Input: part model. Units: mm. Frame: model coordinates. A direction names the side the tool comes from. Give positions to 0.01 mm unless a question says otherwise; leave off trailing zeros. Write each loop counter-clockwise with the first axis right and the second up, starting at its lowest first coordinate (ties: lowest second). Pieces come first, ordered by that corner, then holes. Notation, with made-up numbers: (69, 2.5) - (82, 2.5) arc R18 cw to (82, 20.5) - close; hole circle Ø2 at (43, 1). An arc over 180 degrees is marked (long way). Answer as a JSON object with one key per item and string values. Group by question number.
Autodesk Inventor part; units mm, degrees
ref_plane "YZ Plane" through (0, 0, 0) normal (1, 0, 0) x (0, 1, 0)
ref_plane "XZ Plane" through (0, 0, 0) normal (0, 1, 0) x (-1, 0, 0)
ref_plane "XY Plane" through (0, 0, 0) normal (0, 0, 1) x (1, 0, 0)
sketch "Szkic1" plane through (0, 0, 0) normal (1, 0, 0) x (0, 1, 0)
  line L0 (3.5782, 14) -> (0.5782, 14)
  line L1 (0.5782, 14) -> (0.5782, 23)
  line L2 (0.5782, 23) -> (26.5782, 23)
  arc A0 (49.5782, 0) -> (26.5782, 23) centre (26.5782, 0) ccw
  line L3 (3.5782, 14) -> (3.5782, 18)
  line L4 (3.5782, 18) -> (26.5782, 18)
  arc A1 (44.5782, 0) -> (26.5782, 18) centre (26.5782, 0) ccw
  line L5 (3.5782, -14) -> (0.5782, -14)
  line L6 (0.5782, -14) -> (0.5782, -23)
  line L7 (0.5782, -23) -> (26.5782, -23)
  arc A2 (26.5782, -23) -> (49.5782, 0) centre (26.5782, 0) ccw
  line L8 (3.5782, -14) -> (3.5782, -18)
  line L9 (3.5782, -18) -> (26.5782, -18)
  arc A3 (26.5782, -18) -> (44.5782, 0) centre (26.5782, 0) ccw
  line L10 (51.5782, 6.5) -> (44.5782, 6.5)
  line L11 (44.5782, 6.5) -> (44.5782, -6.5)
  line L12 (44.5782, -6.5) -> (51.5782, -6.5)
  line L13 (54.5782, -3.5) -> (54.5782, 3.5)
  arc A4 (54.5782, 3.5) -> (51.5782, 6.5) centre (51.5782, 3.5) ccw
  arc A5 (51.5782, -6.5) -> (54.5782, -3.5) centre (51.5782, -3.5) ccw
  point P0 (0, 0)
  point P1 (2.0782, 14)
  point P2 (3.5782, 16)
  point P3 (2.0782, -14)
  point P4 (0.5782, 18.5)
  point P5 (48.6406, -6.5)
  point P6 (48.6406, 6.5)
  dimension "d0" = 9
  dimension "d2" = 5
  dimension "d3" = 3
  dimension "d4" = 23
  dimension "d5" = 14
  dimension "d6" = 14
  dimension "d7" = 13
  dimension "d8" = 54
  dimension "d9" = 3
  dimension "d10" = 3
sketch "Szkic2" plane through (0, 0, 0) normal (1, 0, 0) x (0, 1, 0)
  point P0 (0, 0)
extrude "Wyciągnięcie proste1" add sketch "Szkic1" along normal blind 13
fillet "Zaokrąglenie1" radius 3 1 edges at (6.5, 48.6406, -6.5)
fillet "Zaokrąglenie2" radius 3 1 edges at (6.5, 48.6406, 6.5)
sketch "Szkic3" plane through (0, 54.5782, 3.5) normal (0, 1, 0) x (1, 0, 0)
  point P0 (0, 3.5)
  point P1 (6.5, 3.5)
hole "Otwór1" at (6.5, 54.5782, 0) direction (0, -1, 0) diameter 3.242 end through all
1) Cut plane C-C on x = 6.5. Return the cut outline in (y, z), and give its area (3 significant figures).
2) Reachability of faces 4 (the face through (6.409, 39.374, 19.112)), 5 (the face through (6, 15, 18)), 6 (the face through (6, 2, 14)) from +Z, -Z, +X, -X, +Y, -Y: full face, straight path, thin tool, end or side. Return the list, or none.
3) Cut plane A-A on y = 10. Return the cut outline in (x, z), and give its area (3 significant figures).
4) Cut plane D-D on z = -5. Return the cut outline in (x, y).
5) Cut plane B-B on z = 0. Return the cut outline in (x, y).
6) Line query: line 1 along Z through (x, y) = (3.75, 21); line 2 along X through (y, z) = (51, 0); line 3 along Y through (x, z) = (4.25, 16). Output: solid intervals per line, ascending. Write a range as from..to.
7) Pin query (flat end, axial travel): P1, Ø1.5, axis at x = 11, y = 47.5, coming from the +Z side; P2, Ø3, axis at x = 8, z = -13, coming from the +Y side; P3, Ø4.5, axis at x = 6, z = -15, coming from the +Y side. Return the tip coordinate at first contact, or that it passes through.
8) Mould query, pull axis X, two halves, no side actions, for faces 1 (the face through (6.59, 49.11, -7.01)), 2 (the face through (0, 43.5, -6.7)), 3 (the face through (5.13, 49.47, 0.87)). Classes: +X half, -X half, draft (parallel to the pull), parting line (faces both ways), or undercut.
Filled in:
{
 "1": {"outline": "(0.58, -23) - (26.58, -23) arc R23 ccw to (47.99, -8.4) arc R3 cw to (50.78, -6.5) - (51.58, -6.5) arc R3 ccw to (54.58, -3.5) - (54.58, -1.62) - (44.51, -1.62) arc R18 cw to (26.58, -18) - (3.58, -18) - (3.58, -14) - (0.58, -14) - close; (0.58, 14) - (3.58, 14) - (3.58, 18) - (26.58, 18) arc R18 cw to (44.51, 1.62) - (54.58, 1.62) - (54.58, 3.5) arc R3 ccw to (51.58, 6.5) - (50.78, 6.5) arc R3 cw to (47.99, 8.4) arc R23 ccw to (26.58, 23) - (0.58, 23) - close", "area": "640 mm²"},
 "2": {"face 4": "+Z, +X, -X, +Y", "face 5": "+X, -X", "face 6": "+X, -X, -Y"},
 "3": {"outline": "(0, -23) - (13, -23) - (13, -18) - (0, -18) - close; (0, 18) - (13, 18) - (13, 23) - (0, 23) - close", "area": "130 mm²"},
 "4": {"outline": "(0, 43.87) - (13, 43.87) - (13, 54.18) - (0, 54.18) - close"},
 "5": {"outline": "(0, 44.58) - (4.88, 44.58) - (4.88, 54.58) - (0, 54.58) - close; (8.12, 44.58) - (13, 44.58) - (13, 54.58) - (8.12, 54.58) - close"},
 "6": {"line 1": "z = -23..-18, 18..23", "line 2": "x = 0..4.88, 8.12..13", "line 3": "y = 0.58..3.58, 34.82..43.1"},
 "7": {"P1": "stops at z = 11.05", "P2": "stops at y = 46.5", "P3": "stops at y = 45.72"},
 "8": {"face 1": "draft", "face 2": "-X half", "face 3": "undercut"}
}
